from build123d import *

# Parameters (mm, degrees)
F0_R       = 4.5
F1_DEPTH   = 200
F2_R       = 4.5
F3_DEPTH   = 8
F4_R       = 1.5
F5_DEPTH   = 33
F6_SIZE2   = 1.3
F6_SIZE    = 7.3726663655
F6_2_SIZE2 = 1.3
F6_2_SIZE  = 7.3726663655
F6_3_SIZE2 = 1.3
F6_3_SIZE  = 7.3726663655


with BuildPart() as f1:
    # F0 (on Front) → F1 (new body)
    with BuildSketch(Plane.XZ):
        Circle(F0_R)
    extrude(amount=F1_DEPTH)

    # F2 (on face) → F3 (join)
    with BuildSketch(Plane.XZ.offset(200)):
        with BuildLine():
            Line((2.4631588878, 6.9413866261), (-5.1490192915, 5.2666498209))
            ThreePointArc((-5.1490192915, 5.2666498209), (-8.1024719288, 2.5690365204), (-7.2429965996, -1.3375351427))
            Line((-7.2429965996, -1.3375351427), (-1.986542892, -7.0925064215))
            ThreePointArc((-1.986542892, -7.0925064215), (1.8263850745, -8.301464784), (4.7798377118, -5.6038514834))
            Line((4.7798377118, -5.6038514834), (7.1355621835, 1.8258566006))
            ThreePointArc((7.1355621835, 1.8258566006), (6.2760868543, 5.7324282636), (2.4631588878, 6.9413866261))
        make_face()
        Circle(F2_R, mode=Mode.SUBTRACT)
        Circle(F2_R)
    extrude(amount=F3_DEPTH)

    # F4 (on face) → F5 (join)
    with BuildSketch(Plane.XZ.offset(208)):
        with Locations((3.322634217, 3.0348149631)):
            Circle(F4_R)
        with Locations((-4.0512359644, 1.2845182602)):
            Circle(F4_R)
        with Locations((0.9669097453, -4.3948931209)):
            Circle(F4_R)
    extrude(amount=F5_DEPTH)

    # F6
    f6_edges = [f1.edges().sort_by_distance(p)[0] for p in [
        (-0.53309, -241, -4.394893),
    ]]
    f6_side = f1.faces().sort_by_distance((-0.53309, -224.5, -4.394893))[0]
    chamfer(f6_edges, length=F6_SIZE, length2=F6_SIZE2, reference=f6_side)

    # F6#2
    f6_2_edges = [f1.edges().sort_by_distance(p)[0] for p in [
        (-5.551236, -241, 1.284518),
    ]]
    f6_2_side = f1.faces().sort_by_distance((-5.551236, -224.5, 1.284518))[0]
    chamfer(f6_2_edges, length=F6_2_SIZE, length2=F6_2_SIZE2, reference=f6_2_side)

    # F6#3
    f6_3_edges = [f1.edges().sort_by_distance(p)[0] for p in [
        (1.822634, -241, 3.034815),
    ]]
    f6_3_side = f1.faces().sort_by_distance((1.822634, -224.5, 3.034815))[0]
    chamfer(f6_3_edges, length=F6_3_SIZE, length2=F6_3_SIZE2, reference=f6_3_side)


solid = f1.part
The listing builds one solid part. Answer for the finished solid, in the listing's coordinates (mm). A direction names the side the tool comes from. Give positions to 0.01 mm unless a question says otherwise; leave off trailing zeros. Order: outer loops, then holes, each group sorted by start corner. A loop starts at its lowest first (then second) coordinate and runs counter-clockwise, first axis right, second up. Notation, with made-up numbers: (-40, 21) -> (19, 21) arc R22 cw to (19, 38) -> close; hole circle Ø5 at (54.5, 0). An arc over 180 degrees is marked (long way). Put each result on its own line as item: value.
Item 1: A cutting plane is placed at A-A on y = -192. Give the vertices of the cut face in (x, z), plus the area to 3 significant figures.
Established:
outline: circle Ø9 at (0, 0)
area: 63.6 mm^2
Item 2: For faces 1 (the face through (-1, -208, -1)), 2 (the face through (-0.59, -98.6, 4.46)), 3 (the face through (5.94, -203.94, -1.94)), determine the directions among +Z, -Z, +X, -X, +Y, -Y from which every point of the face is accessible in a straight line to the end or side of a thin tool.
Established:
face 1: -Y
face 2: +Y
face 3: -Z, +X, +Y, -Y
Item 3: Given P1, Ø4, axis at x = 5.5, z = -6, coming from the +Y side; P2, Ø8, axis at y = -132, z = -5, coming from the -X side; P3, Ø1, axis at x = -6.5, z = -4.5, coming from the +Y side; P4, Ø3, axis at x = 0.5, y = -192, coming from the +Z side, each flat-ended and moving along its own axis, determine where each tip first touches the part or whether it passes through.
Established:
P1: stops at y = -200
P2: stops at x = -4.39
P3: passes through
P4: stops at z = 4.5
Item 4: Straight lines are drawn through the part: line 1 (Y direction, x = -2.5, z = 5.25); line 2 (Z direction, x = 0, y = -57); line 3 (Y direction, x = -2.75, z = 3.25). For each, find the intervals that lie inside material, in ascending order.
Established:
line 1: y = -208 to -200
line 2: z = -4.5 to 4.5
line 3: y = -208 to 0
